Autodesk Inventor part; units mm, degrees
ref_plane "YZ Plane" through (0, 0, 0) normal (1, 0, 0) x (0, 1, 0)
ref_plane "XZ Plane" through (0, 0, 0) normal (0, 1, 0) x (-1, 0, 0)
ref_plane "XY Plane" through (0, 0, 0) normal (0, 0, 1) x (1, 0, 0)
sketch "Sketch1" plane through (0, 0, 0) normal (0, 1, 0) x (-1, 0, 0)
  line L0 (0, 0) -> (119, 0)
  line L1 (119, 0) -> (119, -90.25)
  line L2 (119, -90.25) -> (0, -90.25)
  line L3 (0, -90.25) -> (0, 0)
  dimension "d0" = 119
  dimension "d1" = 90.25
extrude "Extrusion1" add sketch "Sketch1" along normal blind 3
sketch "Sketch2" plane through (-119, 0, 0) normal (0, 0, 1) x (1, 0, 0)
  line L0 (119, 0) -> (0, 0)
  line L1 (0, 0) -> (119, 0)
  line L2 (119, 0) -> (119, 23)
  line L3 (119, 23) -> (0, 23)
  line L4 (0, 23) -> (0, 0)
  dimension "d4" = 23
extrude "Extrusion2" add sketch "Sketch2" along normal blind 3
sketch "Sketch3" plane through (-119, 23, 0) normal (0, 1, 0) x (1, 0, 0)
  line L0 (119, 0) -> (119, 90.25)
  line L1 (119, 0) -> (0, 0)
  line L2 (0, 0) -> (0, -63)
  line L3 (0, -63) -> (119, -63)
  line L4 (119, -63) -> (119, 0)
  dimension "d7" = 119
  dimension "d8" = 63
extrude "Extrusion3" add sketch "Sketch3" along normal blind 3
fillet "Fillet1" radius 15 2 edges at (-59.5, 26, 0) (-59.5, 23, 3)
sketch "Sketch4" plane through (0, 0, -90.25) normal (0, 0, -1) x (-1, 0, 0)
  line L0 (0, 3) -> (119, 3)
  line L1 (15, 3) -> (25, 3)
  line L2 (25, 3) -> (25, 0)
  line L3 (25, 0) -> (15, 0)
  line L4 (15, 0) -> (15, 3)
  line L5 (0, 0) -> (0, 3)
  line L6 (94, 3) -> (104, 3)
  line L7 (104, 3) -> (104, 0)
  line L8 (104, 0) -> (94, 0)
  line L9 (94, 0) -> (94, 3)
  line L10 (119, 0) -> (119, 3)
  point P0 (15, 1.5)
  point P1 (0, 1.5)
  point P2 (104, 1.5)
  point P3 (119, 1.5)
  dimension "d12" = 10
  dimension "d13" = 3
  dimension "d14" = 15
  dimension "d15" = 10
  dimension "d16" = 3
  dimension "d17" = 15
extrude "Extrusion4" add sketch "Sketch4" along normal blind 10
sketch "Sketch5" plane through (-119, 23, 63) normal (0, 0, 1) x (1, 0, 0)
  line L0 (0, 3) -> (119, 3)
  line L1 (15, 3) -> (25, 3)
  line L2 (25, 3) -> (25, 0)
  line L3 (25, 0) -> (15, 0)
  line L4 (15, 0) -> (15, 3)
  line L5 (94, 3) -> (104, 3)
  line L6 (104, 3) -> (104, 0)
  line L7 (104, 0) -> (94, 0)
  line L8 (94, 0) -> (94, 3)
  line L9 (0, 0) -> (0, 3)
  line L10 (119, 0) -> (119, 3)
  point P0 (119, -23)
  point P1 (15, 1.5)
  point P2 (0, 1.5)
  point P3 (119, 1.5)
  point P4 (104, 1.5)
  point P5 (104, 3)
  point P6 (94, 3)
  point P7 (25, 3)
  dimension "d20" = 10
  dimension "d21" = 3
  dimension "d22" = 10
  dimension "d23" = 3
  dimension "d24" = 15
  dimension "d25" = 15
extrude "Extrusion5" add sketch "Sketch5" along normal blind 10
sketch "Sketch6" plane through (-119, 26, 0) normal (0, 1, 0) x (1, 0, 0)
  circle A0 centre (20, -68) radius 1.65
  line L0 (15, -63) -> (15, -73)
  line L1 (25, -73) -> (15, -73)
  circle A1 centre (99, -68) radius 1.65
  line L2 (104, -73) -> (94, -73)
  line L3 (94, -63) -> (94, -73)
  point P0 (119, 0)
  point P1 (15, -68)
  point P2 (99, -73)
  dimension "d28" = 3.3
  dimension "d29" = 5
  dimension "d30" = 5
  dimension "d31" = 3.3
  dimension "d32" = 5
  dimension "d33" = 5
extrude "Extrusion6" cut sketch "Sketch6" against normal blind 5
sketch "Sketch7" plane through (0, 3, 0) normal (0, 1, 0) x (1, 0, 0)
  circle A0 centre (-99, 95.25) radius 1.65
  circle A1 centre (-20, 95.25) radius 1.65
  line L0 (-104, 90.25) -> (-104, 100.25)
  line L1 (-104, 100.25) -> (-94, 100.25)
  line L2 (-25, 90.25) -> (-25, 100.25)
  line L3 (-25, 100.25) -> (-15, 100.25)
  point P0 (0, 0)
  point P1 (-104, 95.25)
  dimension "d36" = 3.3
  dimension "d37" = 3.3
  dimension "d38" = 5
  dimension "d39" = 5
  dimension "d40" = 5
  dimension "d41" = 5
extrude "Extrusion7" cut sketch "Sketch7" against normal blind 5
fillet "Fillet2" radius 5 16 edges at (-15, 24.5, 73) (-15, 24.5, 63) (-25, 24.5, 73) (-25, 24.5, 63) (-104, 24.5, 63) (-104, 24.5, 73) (-94, 24.5, 73) (-94, 24.5, 63) (-15, 1.5, -90.25) (-15, 1.5, -100.25) (-25, 1.5, -100.25) (-25, 1.5, -90.25) (-94, 1.5, -100.25) (-104, 1.5, -100.25) (-104, 1.5, -90.25) (-94, 1.5, -90.25)
fillet "Fillet3" radius 2 4 edges at (0, 1.5, -90.25) (-119, 1.5, -90.25) (-119, 24.5, 63) (0, 24.5, 63)
sketch "Sketch8" plane through (0, 3, 0) normal (0, 1, 0) x (1, 0, 0)
  line L0 (-37, 6.25) -> (-12, 6.25)
  line L1 (-12, 6.25) -> (-12, 77.25)
  line L2 (-12, 77.25) -> (-37, 77.25)
  line L3 (-37, 77.25) -> (-37, 6.25)
  line L4 (0, 0) -> (0, 88.25)
  line L5 (-2, 90.25) -> (-10, 90.25)
  dimension "d46" = 25
  dimension "d47" = 71
  dimension "d48" = 12
  dimension "d49" = 13
extrude "Extrusion8" cut sketch "Sketch8" against normal blind 5
equation "\"d34\" = d30"
equation "\"d42\" = d30"
equation "\"d50\" = d30"
properties part number "top"
Here's how the part is built. I have some questions about the finished solid (model axes, mm). A direction names the side the tool comes from. Coordinates: 2 decimals unless noted, no trailing zeros. Write each loop counter-clockwise with the first axis right and the second up, starting at its lowest first coordinate (ties: lowest second). Pieces come first, ordered by that corner, then holes. Notation, with made-up numbers: (59, -14.75) -> (79, -14.75) arc R25 ccw to (79, 3.25) -> close; hole circle Ø11 at (11, 88.25). An arc over 180 degrees is marked (long way). Use a Markdown table: item, result. Add a question column.
(1) Please list where these lines run through material, in increasing order: line 1 (X direction, y = 25, z = 68); line 2 (Z direction, x = -20, y = 1); line 3 (Y direction, x = -70, z = -40).
(2) We'd pull the mould along Z, two halves only. Please class faces 1 (the flat face through (-119, 2, -14)), 2 (the cylindrical face through (-20.4, 24.5, 69.6)), 3 (the cylindrical face through (-60.33, 21.72, 4.51)), 4 (the cylindrical face through (-100.31, 1.52, -94.25)): +Z half, -Z half, draft (parallel to the pull), parting line (faces both ways), or undercut.
(3) If we section it at B-B, the plane z = -82.5: Write out the boundary of the cut face in (x, y).
(4) For faces 5 (the flat face through (-60, 23, 39)), 6 (the cylindrical face through (-95.43, 1.52, -98.75)), 7 (the flat face through (-72, 3, -49)), which set-ups out of +Z, -Z, +X, -X, +Y, -Y let a thin tool reach every point of the face, with its end or its side?
(5) If we section it at C-C, the plane y = 17.5: Write out the boundary of the cut face in (x, z).
(6) I'm going to push flat-ended pins straight in: P1, Ø0.9, axis at x = -7.5, y = 25, coming from the +Z side; P2, Ø10, axis at x = -27.5, z = 8.5, coming from the +Y side; P3, Ø6.5, axis at x = -79, y = 2, coming from the +Z side; P4, Ø0.9, axis at y = 1, z = -49.5, coming from the +X side. Where does each tip first touch, or does it pass through?
(7) If we section it at A-A, the plane x = -43.5: Write out the boundary of the cut face in (y, z), and give its area (3 significant figures).
Outcome:
| question | item | result |
|---|---|---|
| 1 | line 1 | x = -104 to -100.65, -97.35 to -94, -25 to -21.65, -18.35 to -15 |
| 1 | line 2 | z = -100.25 to -96.9, -93.6 to -77.25, -6.25 to 3 |
| 1 | line 3 | y = 0 to 3 |
| 2 | face 1 | draft |
| 2 | face 2 | undercut |
| 2 | face 3 | -Z half |
| 2 | face 4 | undercut |
| 3 | outline | (-119, 0) -> (0, 0) -> (0, 3) -> (-119, 3) -> close |
| 4 | face 5 | +Z, +X, -X, -Y |
| 4 | face 6 | -Z, +Y, -Y |
| 4 | face 7 | -Z, +X, -X, +Y |
| 5 | outline | (-119, 1.48) -> (0, 1.48) -> (0, 6.39) -> (-119, 6.39) -> close |
| 6 | P1 | stops at z = 63 |
| 6 | P2 | stops at y = 25.92 |
| 6 | P3 | stops at z = 3 |
| 6 | P4 | stops at x = 0 |
| 7 | outline | (0, -90.25) -> (3, -90.25) -> (3, 0) -> (11, 0) arc R15 ccw to (26, 15) -> (26, 63) -> (23, 63) -> (23, 18) arc R15 cw to (8, 3) -> (0, 3) -> close |
| 7 | area | 529 mm^2 |
